Here's how the part is built. I have some questions about the finished solid (model axes, mm). A direction names the side the tool comes from. Round coordinates to 2 decimals unless told otherwise and drop trailing zeros. Order: outer loops, then holes, each group sorted by start corner. A loop starts at its lowest first (then second) coordinate and runs counter-clockwise, first axis right, second up. Notation, with made-up numbers: (9.5, -8.5) -> (34.5, -8.5) arc R19 cw to (34.5, 5.5) -> close; hole circle Ø5 at (64, 12). An arc over 180 degrees is marked (long way). Use a Markdown table: item, result. Add a question column.
from build123d import *

# Parameters (mm, degrees)
ESQUISSE1_R             = 5
BOSS_EXTRU_1_DEPTH      = 85
ESQUISSE3_R             = 5
ESQUISSE3_R_2           = 4
BOSS_EXTRU_2_DEPTH      = 15
ESQUISSE4_R             = 3.5
ESQUISSE4_R_2           = 2
ENL_V_MAT_EXTRU_1_DEPTH = 28
ESQUISSE6_R             = 5.5
ENL_V_MAT_EXTRU_2_DEPTH = 5.5


with BuildPart() as part:
    # Esquisse1 → Boss.-Extru.1 (new body)
    with BuildSketch(Plane.XY):
        Polygon((-55.609176617, 28), (-44, 18), (-44, -42), (-86.5, -84.5), (-86.5, -109.5), (-76.5, -119.5), (-16.5, -119.5), (46, -57), (46, 28), (66, 28), (66, 41), (64, 43), (-82, 43), (-84, 41), (-84, 28), align=None)
        with Locations((-64, -97)):
            Circle(ESQUISSE1_R, mode=Mode.SUBTRACT)
    extrude(amount=-BOSS_EXTRU_1_DEPTH)

    # Esquisse3 → Boss.-Extru.2 (add)
    with BuildSketch(Plane.XY):
        Circle(ESQUISSE3_R)
        with Locations((0, 26)):
            Circle(ESQUISSE3_R_2)
    extrude(amount=BOSS_EXTRU_2_DEPTH)

    # Esquisse4 → Enlèv. mat.-Extru.1 (cut)
    with BuildSketch(Plane(origin=(0, 43, 0), x_dir=(1, 0, 0), z_dir=(0, 1, 0))):
        with Locations((-74, 70)):
            Circle(ESQUISSE4_R)
        with Locations((-74, 42.5)):
            Circle(ESQUISSE4_R_2)
        with Locations((-74, 15)):
            Circle(ESQUISSE4_R)
    enl_v_mat_extru_1 = extrude(amount=-ENL_V_MAT_EXTRU_1_DEPTH, mode=Mode.SUBTRACT)

    # Esquisse6 → Enlèv. mat.-Extru.2 (cut)
    with BuildSketch(Plane(origin=(0, 43, 0), x_dir=(1, 0, 0), z_dir=(0, 1, 0))):
        with Locations((-74, 70)):
            Circle(ESQUISSE6_R)
        with Locations((-74, 15)):
            Circle(ESQUISSE6_R)
    enl_v_mat_extru_2 = extrude(amount=-ENL_V_MAT_EXTRU_2_DEPTH, mode=Mode.SUBTRACT)

    # Symétrie1: Enlèv. mat.-Extru.1, Enlèv. mat.-Extru.2 across plane
    add(enl_v_mat_extru_1.mirror(Plane(origin=(-9, 0, 0), x_dir=(0, 0, 1), z_dir=(1, 0, 0))), mode=Mode.SUBTRACT)
    add(enl_v_mat_extru_2.mirror(Plane(origin=(-9, 0, 0), x_dir=(0, 0, 1), z_dir=(1, 0, 0))), mode=Mode.SUBTRACT)


solid = part.part
(1) I want a section at B-B on x = 56. List the corners of the cut face in (y, z) for me, and give its area (3 significant figures).
(2) I want a section at C-C on x = -74. List the corners of the cut face in (y, z) for me.
(3) On a 3-axis mill with a long thin cutter (end or side, diameter ignored), from which of +Z, -Z, +X, -X, +Y, -Y can I reach the whole of each face in a straight line? I mean faces 1 (the flat face through (53.6, 28, -41.9)), 2 (the flat face through (-86.5, -97, -42)), 3 (the flat face through (52, 37.5, -70)), 4 (the flat face through (-70, 28, -42)), 5 (the cylindrical face through (-1.08, -4.88, 7.4)). Say none if no direction works.
(4) I'm going to push flat-ended pins straight in: P1, Ø1, axis at y = 0, z = -61, coming from the -X side; P2, Ø14.5, axis at x = 56, z = -70, coming from the -Y side; P3, Ø1, axis at x = 14, y = 7, coming from the +Z side. Where does each tip first touch, or does it pass through?
(5) I want a section at A-A on z = -15. State how many separate pieces and enclosed holes the cut face has, and give its area (3 significant figures).
(6) I want a section at D-D on y = 0. List the corners of the cut face in (x, z) for me, and give its area (3 significant figures).
(7) Please list where these lines run through material, in increasing order: probe 1 along Z at (x, y) = (-74, 32); probe 2 along Z at (x, y) = (-74, 41); probe 3 along X at (y, z) = (40, -70). Write a range as from..to.
(8) If we mould it in two halves opening along Y, with no side actions, what happens to faces 6 (the flat face through (-47, -119.5, -42)), 7 (the cylindrical face through (59.497, 32.817, -15.154)), 8 (the cylindrical face through (-0.521, 29.966, 7.395))? For each: pulls with the +Y half, pulls with the -Y half, needs draft (parallel to the pull), parting line crosses it, or undercut.
Output:
| question | item | result |
|---|---|---|
| 1 | outline | (28, -85) -> (43, -85) -> (43, -75.5) -> (37.5, -75.5) -> (37.5, -73.5) -> (28, -73.5) -> close; (28, -66.5) -> (37.5, -66.5) -> (37.5, -64.5) -> (43, -64.5) -> (43, -44.5) -> (28, -44.5) -> close; (28, -40.5) -> (43, -40.5) -> (43, -20.5) -> (37.5, -20.5) -> (37.5, -18.5) -> (28, -18.5) -> close; (28, -11.5) -> (37.5, -11.5) -> (37.5, -9.5) -> (43, -9.5) -> (43, 0) -> (28, 0) -> close |
| 1 | area | 961 mm² |
| 2 | outline | (-119.5, -85) -> (-72, -85) -> (-72, 0) -> (-119.5, 0) -> close; (28, -85) -> (43, -85) -> (43, -75.5) -> (37.5, -75.5) -> (37.5, -73.5) -> (28, -73.5) -> close; (28, -66.5) -> (37.5, -66.5) -> (37.5, -64.5) -> (43, -64.5) -> (43, -44.5) -> (28, -44.5) -> close; (28, -40.5) -> (43, -40.5) -> (43, -20.5) -> (37.5, -20.5) -> (37.5, -18.5) -> (28, -18.5) -> close; (28, -11.5) -> (37.5, -11.5) -> (37.5, -9.5) -> (43, -9.5) -> (43, 0) -> (28, 0) -> close |
| 3 | face 1 | +Z, -Z, +X, -Y |
| 3 | face 2 | +Z, -Z, -X, +Y, -Y |
| 3 | face 3 | +Y |
| 3 | face 4 | +Z, -Z, -X |
| 3 | face 5 | +Z |
| 4 | P1 | x = -44 |
| 4 | P2 | y = 28 |
| 4 | P3 | z = 0 |
| 5 | separate pieces | 3 |
| 5 | enclosed holes | 1 |
| 5 | area | 15,600 mm² |
| 6 | outline | (-44, -85) -> (46, -85) -> (46, 0) -> (5, 0) -> (5, 15) -> (-5, 15) -> (-5, 0) -> (-44, 0) -> close |
| 6 | area | 7,800 mm² |
| 7 | probe 1 | -85..-73.5, -66.5..-44.5, -40.5..-18.5, -11.5..0 |
| 7 | probe 2 | -85..-75.5, -64.5..-44.5, -40.5..-20.5, -9.5..0 |
| 7 | probe 3 | -84..-79.5, -68.5..50.5, 61.5..66 |
| 8 | face 6 | pulls with the -Y half |
| 8 | face 7 | needs draft |
| 8 | face 8 | undercut |
